The model under review builds one solid part; all positions refer to its coordinate system, in mm. A direction names the side the tool comes from. Coordinates: 2 decimals unless noted, no trailing zeros. Order: outer loops, then holes, each group sorted by start corner. A loop starts at its lowest first (then second) coordinate and runs counter-clockwise, first axis right, second up. Notation, with made-up numbers: M 5,-1.5 L 36,-1.5 A29 ccw 36,27.5 Z; hole C 25.25,7.25 d11. An arc over 180 degrees is marked long. One line per item, written item: value.
Autodesk Inventor part; units mm, degrees
ref_plane "YZ Plane" through (0, 0, 0) normal (1, 0, 0) x (0, 1, 0)
ref_plane "XZ Plane" through (0, 0, 0) normal (0, 1, 0) x (-1, 0, 0)
ref_plane "XY Plane" through (0, 0, 0) normal (0, 0, 1) x (1, 0, 0)
sketch "Sketch1" plane through (0, 0, 0) normal (0, 0, 1) x (1, 0, 0)
  line L0 (-357.1541, -65.4988) -> (-437.5068, -65.4988) construction
  line L1 (-357.1541, -65.4988) -> (-357.1541, -57.4988) construction
  line L2 (-357.1541, -57.4988) -> (-403.5317, -57.4988) construction
  line L3 (-415.2682, -47.6507) -> (-403.5317, -57.4988) construction
  line L4 (-415.2682, -47.6507) -> (-435.2333, 65.5771) construction
  line L5 (-431.1016, 70.5012) -> (-435.2333, 65.5771) construction
  line L6 (-431.1016, 70.5012) -> (-418.2505, 70.5012) construction
  line L7 (-418.2505, 70.5012) -> (-418.2505, 78.5012) construction
  line L8 (-518.2505, 78.5012) -> (-418.2505, 78.5012) construction
  line L9 (-518.2505, 78.5012) -> (-518.2505, 75.5012) construction
  line L10 (-518.2505, 75.5012) -> (-467.3689, 75.5012) construction
  line L11 (-461.5006, 70.5771) -> (-467.3689, 75.5012) construction
  line L12 (-461.5006, 70.5771) -> (-437.5068, -65.4988) construction
  line L13 (4.0058, -65.4988) -> (-76.3469, -65.4988) construction
  line L14 (4.0058, -65.4988) -> (27.9996, 70.5771) construction
  line L15 (33.8679, 75.5012) -> (27.9996, 70.5771) construction
  line L16 (33.8679, 75.5012) -> (84.7495, 75.5012) construction
  line L17 (84.7495, 75.5012) -> (84.7495, 78.5012) construction
  line L18 (-15.2505, 78.5012) -> (84.7495, 78.5012) construction
  line L19 (-15.2505, 78.5012) -> (-15.2505, 70.5012) construction
  line L20 (-15.2505, 70.5012) -> (-2.3994, 70.5012) construction
  line L21 (1.7323, 65.5771) -> (-2.3994, 70.5012) construction
  line L22 (1.7323, 65.5771) -> (-18.2328, -47.6507) construction
  line L23 (-29.9693, -57.4988) -> (-18.2328, -47.6507) construction
  line L24 (-29.9693, -57.4988) -> (-76.3469, -57.4988) construction
  line L25 (-76.3469, -57.4988) -> (-76.3469, -65.4988) construction
  line L26 (-357.1541, -67.4988) -> (-357.1541, -65.4988) construction
  line L27 (-357.1541, -65.4988) -> (-437.5068, -65.4988) construction
  line L28 (-437.5068, -65.4988) -> (-437.1541, -67.4988) construction
  line L29 (-437.1541, -67.4988) -> (-357.1541, -67.4988) construction
  line L30 (3.6531, -67.4988) -> (4.0058, -65.4988) construction
  line L31 (4.0058, -65.4988) -> (-76.3469, -65.4988) construction
  line L32 (-76.3469, -65.4988) -> (-76.3469, -67.4988) construction
  line L33 (-76.3469, -67.4988) -> (3.6531, -67.4988) construction
  line L34 (-416.865, -38.5948) -> (-16.636, -38.5948)
  line L35 (-16.636, -38.5948) -> (-18.2328, -47.6507)
  line L36 (-18.2328, -47.6507) -> (-29.9693, -57.4988)
  line L37 (-29.9693, -57.4988) -> (-76.3469, -57.4988)
  line L38 (-76.3469, -57.4988) -> (-76.3469, -67.4988)
  line L39 (-76.3469, -67.4988) -> (-357.1541, -67.4988)
  line L40 (-357.1541, -67.4988) -> (-357.1541, -57.4988)
  line L41 (-357.1541, -57.4988) -> (-403.5317, -57.4988)
  line L42 (-403.5317, -57.4988) -> (-415.2682, -47.6507)
  line L43 (-415.2682, -47.6507) -> (-416.865, -38.5948)
extrude "Extrusion1" add sketch "Sketch1" against normal blind 32
sketch "Sketch2" plane through (0, 0, 0) normal (0, 0, 1) x (1, 0, 0)
  line L0 (3.6531, -67.4988) -> (4.0058, -65.4988)
  line L1 (4.0058, -65.4988) -> (-66.3469, -65.4988)
  line L2 (-66.3469, -65.4988) -> (-66.3469, -67.4988)
  line L3 (-66.3469, -67.4988) -> (3.6531, -67.4988)
  line L4 (4.0058, -65.4988) -> (-66.3469, -65.4988)
  line L5 (4.0058, -65.4988) -> (27.118, 65.5771)
  line L6 (-15.2505, 78.5012) -> (-15.2505, 72.5012)
  line L7 (1.7323, 65.5771) -> (-18.5801, -49.6204)
  line L8 (-66.3469, -59.4988) -> (-66.3469, -65.4988)
  line L9 (-367.1541, -65.4988) -> (-437.5068, -65.4988)
  line L10 (-367.1541, -65.4988) -> (-367.1541, -59.4988)
  line L11 (-414.9209, -49.6204) -> (-435.2333, 65.5771)
  line L12 (-418.2505, 72.5012) -> (-418.2505, 78.5012)
  line L13 (-460.619, 65.5771) -> (-437.5068, -65.4988)
  line L14 (-367.1541, -67.4988) -> (-367.1541, -65.4988)
  line L15 (-367.1541, -65.4988) -> (-437.5068, -65.4988)
  line L16 (-437.5068, -65.4988) -> (-437.1541, -67.4988)
  line L17 (-437.1541, -67.4988) -> (-367.1541, -67.4988)
  line L18 (-357.1541, -57.4988) -> (-66.3469, -57.4988)
  line L19 (-66.3469, -57.4988) -> (-66.3469, -67.4988)
  line L20 (-66.3469, -67.4988) -> (-357.1541, -67.4988)
  line L21 (-357.1541, -67.4988) -> (-357.1541, -57.4988)
  line L22 (1.7323, 65.5771) -> (-4.0776, 72.5012)
  line L23 (-429.4234, 72.5012) -> (-435.2333, 65.5771)
  line L24 (35.3697, 72.5012) -> (27.118, 65.5771)
  line L25 (84.7495, 72.5012) -> (84.7495, 78.5012)
  line L26 (-518.2505, 78.5012) -> (-518.2505, 72.5012)
  line L27 (-460.619, 65.5771) -> (-468.8707, 72.5012)
  line L28 (-15.2505, 78.5012) -> (84.7495, 78.5012)
  line L29 (-518.2505, 78.5012) -> (-418.2505, 78.5012)
  line L30 (-66.3469, -59.4988) -> (-30.3528, -59.4988)
  line L31 (84.7495, 72.5012) -> (35.3697, 72.5012)
  line L32 (-4.0776, 72.5012) -> (-15.2505, 72.5012)
  line L33 (-30.3528, -59.4988) -> (-18.5801, -49.6204)
  line L34 (-414.9209, -49.6204) -> (-403.1482, -59.4988)
  line L35 (-418.2505, 72.5012) -> (-429.4234, 72.5012)
  line L36 (-468.8707, 72.5012) -> (-518.2505, 72.5012)
  line L37 (-403.1482, -59.4988) -> (-367.1541, -59.4988)
  point P0 (0, 0)
extrude "Extrusion2" add sketch "Sketch2" against normal up to surface (32 mm away) contours L20 L21 L18 L19 L8 L2
chamfer "Chamfer1" distance 2 angle 45 2 edges at (-216.7505, -67.4988, -32) (-216.7505, -67.4988, 0)
properties part number "DNW_CON" material "Wood (Birch)"
(1) We need section A-A, the plane z = -25. State the section outline as (x, y) points (3 decimals).
Geometry results:
outline: M -416.865,-38.595 L -415.268,-47.651 L -403.532,-57.499 L -357.154,-57.499 L -357.154,-67.499 L -66.347,-67.499 L -66.347,-57.499 L -29.969,-57.499 L -18.233,-47.651 L -16.636,-38.595 Z
(2) We need section C-C, the plane y = -61. State the section outline as (x, z) points, plus the area to 3 significant figures.
Geometry results:
outline: M -357.15,-32 L -66.35,-32 L -66.35,0 L -357.15,0 Z
area: 9,310 mm2
(3) Insertion check: pin 1 Ø5 at (y, z) = (-60.5, -17) entering from -X; pin 2 Ø1.5 at (x, z) = (-362, -11) entering from -Y; pin 3 Ø8 at (y, z) = (-44.5, -4) entering from +X. Each pin has a flat end and moves straight along its axis. Give the tip position at first contact, or say it passes through.
Geometry results:
pin 1: stops at x = -357.15
pin 2: stops at y = -57.5
pin 3: stops at x = -16.97
(4) Tool access review of faces 1 (the flat face through (-220, -38.595, -16)), 2 (the flat face through (-66.347, -62, -16)), 3 (the flat face through (-380, -57.499, -16)): name each direction out of +Z, -Z, +X, -X, +Y, -Y from which nothing blocks a thin tool from reaching the whole face with its end or side.
Geometry results:
face 1: +Z, -Z, +X, -X, +Y
face 2: +Z, -Z, +X, -Y
face 3: +Z, -Z, -X, -Y
(5) For L1, parallel to Y at x = -381, z = -26; L2, parallel to X at y = -61.5, z = -26.5; L3, parallel to X at y = -52, z = -28, list the stretches that pass through material, from the lowest coordinate up.
Geometry results:
L1: y = -57.5 to -38.59
L2: x = -357.15 to -66.35
L3: x = -410.08 to -23.42
(6) We need section B-B, the plane x = -51. State the section outline as (y, z) points, plus the area to 3 significant figures.
Geometry results:
outline: M -57.5,-32 L -38.59,-32 L -38.59,0 L -57.5,0 Z
area: 605 mm2
